For this review, take the finished solid that the model builds, in its own axes (mm). A direction names the side the tool comes from. Round coordinates to 2 decimals unless told otherwise and drop trailing zeros. Write each loop counter-clockwise with the first axis right and the second up, starting at its lowest first coordinate (ties: lowest second). Pieces come first, ordered by that corner, then holes. Notation, with made-up numbers: (48, 20.5) -> (80, 20.5) arc R15 cw to (80, 42.5) -> close; hole circle Ø11 at (49, -18). An arc over 180 degrees is marked (long way). Write each question's results on one line, items separated by ' | '. Start each with the question number.
Item 1: The part is to be moulded in two halves that separate along Z. For faces 4 (the flat face through (-1, -25, -7)), 5 (the cylindrical face through (2.47, -24.72, 6.85)), 6 (the flat face through (1.85, -12.32, 10.39)), say which applies: +Z half, -Z half, draft (parallel to the pull), parting line (faces both ways), or undercut.
Item 2: To check wall thickness, follow line 1 along Z through (x, y) = (-8.5, -18); line 2 along Z through (x, y) = (-8.25, -22); line 3 along X through (y, z) = (-18, -1). State the ranges of each line that lie inside material, in increasing order.
Item 3: Tool access review of faces 1 (the flat face through (4.5, -12.32, 11.28)), 2 (the flat face through (-1.621, -12, 3)), 3 (the flat face through (0, -12, 1)): name each direction out of +Z, -Z, +X, -X, +Y, -Y from which nothing blocks a thin tool from reaching the whole face with its end or side.
Item 4: Add section A-A (z = 9.5). State the section outline as (x, y) points.
Item 5: Add section C-C (x = -12.25). State the section outline as (y, z) points.
Item 6: Clearance check with flat-ended pins moving along their axes: pin 1 (7.5 mm diameter, centred on y = -12, z = -2, fed in from -X); pin 2 (8 mm diameter, centred on x = -5, y = -16, fed in from +Z); pin 3 (6 mm diameter, centred on x = -10.5, y = -19, fed in from +Z). State where each tip first meets the part, or that it passes through.
Item 7: Add section D-D (z = -2). State the section outline as (x, y) points.
from build123d import *

# Parameters (mm, degrees)
F1_DEPTH       = 25
F2_R           = 1.5
F4_D           = 4.4
F4_CSINK_D     = 8.96
F4_CSINK_ANGLE = 90


with BuildPart() as f1:
    # F0 (on Front) → F1 (new body)
    with BuildSketch(Plane.XZ):
        Polygon((0, -20.1055445863), (0, -13.0393103669), (0, 14.3368082835), (2, 14.3368082835), (1.7, 6.3368082835), (3.6758784442, 6.0271239706), (5.3791421656, 16.8944554137), (-1.6208578344, 16.8944554137), (-1.6208578344, -10.1055445863), (-11.6208578344, -10.1055445863), (-14.5, -20.1055445863), align=None)
    extrude(amount=F1_DEPTH)

    # F2
    f2_edges = [f1.edges().sort_by_distance(p)[0] for p in [
        (-1.620858, -12.5, 16.894455),
        (5.379142, -12.5, 16.894455),
        (0, -12.5, -20.105545),
        (2.687939, -25, 6.181966),
        (3.675878, -12.5, 6.027124),
    ]]
    fillet(f2_edges, radius=F2_R)

    # F4 (through all)
    with Locations(Plane.YZ):
        with Locations((-7, -14.1055445863), (-18, -14.1055445863)):
            CounterSinkHole(F4_D / 2, F4_CSINK_D / 2, counter_sink_angle=F4_CSINK_ANGLE)


solid = f1.part
Responses:
1) face 4: draft | face 5: -Z half | face 6: undercut
2) line 1: z = -20.11 to -16.31, -11.91 to -10.11 | line 2: z = -20.11 to -10.11 | line 3: x = -1.62 to 0
3) face 1: -Z, +X, +Y, -Y | face 2: +Z, -X, +Y, -Y | face 3: -Z, +Y, -Y
4) outline: (-1.62, -25) -> (0, -25) -> (0, 0) -> (-1.62, 0) -> close; (1.82, -25) -> (4.22, -25) -> (4.22, 0) -> (1.82, 0) -> close
5) outline: (-25, -20.11) -> (0, -20.11) -> (0, -12.29) -> (-5.76, -12.29) arc R2.2 cw (long way) to (-8.24, -12.29) -> (-16.76, -12.29) arc R2.2 cw (long way) to (-19.24, -12.29) -> (-25, -12.29) -> close
6) pin 1: stops at x = -1.62 | pin 2: stops at z = 16.61 | pin 3: stops at z = -10.11
7) outline: (-1.62, -25) -> (0, -25) -> (0, 0) -> (-1.62, 0) -> close
